from build123d import *

# Parameters (mm, degrees)
ESBO_O1_W                = 8.5
ESBO_O1_H                = 27
RESSALTO_EXTRUS_O1_DEPTH = 13
ESBO_O3_R                = 8.3
CORTE_EXTRUS_O1_DEPTH    = 3
ESBO_O4_R                = 6.3
CORTE_EXTRUS_O2_DEPTH    = 5
ESBO_O7_R                = 8.3
CORTE_EXTRUS_O3_DEPTH    = 0.7
ESBO_O8_R                = 2
CORTE_EXTRUS_O4_DEPTH    = 14


with BuildPart() as part:
    # Esboço1 → Ressalto-extrusão1 (new body)
    with BuildSketch(Plane.XY):
        with Locations((4.75, 202.468429513)):
            Rectangle(ESBO_O1_W, ESBO_O1_H)
    extrude(amount=RESSALTO_EXTRUS_O1_DEPTH)

    # Esboço3 → Corte-extrusão1 (cut)
    with BuildSketch(Plane(origin=(9, 0, 0), x_dir=(0, 0, -1), z_dir=(1, 0, 0))):
        with Locations((0, 202.468429513)):
            Circle(ESBO_O3_R)
    extrude(amount=-CORTE_EXTRUS_O1_DEPTH, mode=Mode.SUBTRACT)

    # Esboço4 → Corte-extrusão2 (cut)
    with BuildSketch(Plane(origin=(6, 0, 0), x_dir=(0, 0, -1), z_dir=(1, 0, 0))):
        with Locations((0, 202.468429513)):
            Circle(ESBO_O4_R)
    extrude(amount=-CORTE_EXTRUS_O2_DEPTH, mode=Mode.SUBTRACT)

    # Esboço7 → Corte-extrusão3 (cut)
    with BuildSketch(Plane.ZY.offset(-0.5)):
        with Locations((0, 202.468429513)):
            Circle(ESBO_O7_R)
    extrude(amount=-CORTE_EXTRUS_O3_DEPTH, mode=Mode.SUBTRACT)

    # Esboço8 → Corte-extrusão4 (cut, through all)
    with BuildSketch(Plane.XY.offset(13)):
        with Locations((4.75, 191.968429513)):
            Circle(ESBO_O8_R)
        with Locations((4.75, 212.968429513)):
            Circle(ESBO_O8_R)
    extrude(amount=-CORTE_EXTRUS_O4_DEPTH, mode=Mode.SUBTRACT)


solid = part.part
Model file for the job. Use its own axes, mm. A direction names the side the tool comes from. Coordinates: 2 decimals unless noted, no trailing zeros. Order: outer loops, then holes, each group sorted by start corner. A loop starts at its lowest first (then second) coordinate and runs counter-clockwise, first axis right, second up. Notation, with made-up numbers: (12.5, -28.75) -> (51.5, -28.75) arc R33 cw to (51.5, 6.25) -> close; hole circle Ø9 at (23.5, -23). An arc over 180 degrees is marked (long way). Return JSON: item names as keys, results as strings. Group by question number.
Item 1: Saw through at B-B on x = 4.75. Write the cut outline in (y, z).
Item 2: Wall check: line 1 along Y through (x, z) = (4.75, 8.5); line 2 along Y through (x, z) = (5.25, 10.5); line 3 along Y through (x, z) = (7, 5.75). Give the ranges that are in metal, low to high. Write a range as [from, to].
Item 3: Saw through at C-C on z = 8. Write the cut outline in (x, y), then the cut area to 3 significant figures.
Item 4: Tool access for faces 4 (the cylindrical face through (0.8, 202.3, 8.3)), 5 (the flat face through (2.8, 193.4, 0)), 6 (the cylindrical face through (7.52, 202.65, 8.3)): list every direction of +Z, -Z, +X, -X, +Y, -Y with a clear straight run to the whole face (end or side of a thin tool).
Item 5: Saw through at A-A on z = 1. Write the cut outline in (x, y), then the cut area to 3 significant figures.
Item 6: Flat gauge pins, fed straight in: P1, Ø4, axis at y = 203, z = 5, coming from the +X side; P2, Ø4, axis at y = 198.5, z = 4.5, coming from the -X side; P3, Ø2.5, axis at x = 4.75, y = 191.97, coming from the -Z side; P4, Ø3, axis at x = 6.5, y = 205, coming from the -Z side. Where does each tip first touch, or does it go through?
Item 7: Saw through at D-D on y = 201.5. Write the cut outline in (x, z).
Item 8: Pull direction X, two halves, no side cores. Call faces 1 (the flat face through (1.2, 203, 7)), 2 (the cylindrical face through (5.673, 190.194, 6.591)), 3 (the flat face through (5, 188.968, 6)): pulls with the +X half, pulls with the -X half, needs draft (parallel to the pull), parting line crosses it, or undercut.
Values found:
{
 "1": {"outline": "(188.97, 0) -> (189.97, 0) -> (189.97, 13) -> (188.97, 13) -> close; (193.97, 0) -> (196.17, 0) arc R6.3 cw to (208.77, 0) -> (210.97, 0) -> (210.97, 13) -> (193.97, 13) -> close; (214.97, 0) -> (215.97, 0) -> (215.97, 13) -> (214.97, 13) -> close"},
 "2": {"line 1": "y = [188.97, 189.97], [193.97, 210.97], [214.97, 215.97]", "line 2": "y = [188.97, 190.03], [193.9, 211.03], [214.9, 215.97]", "line 3": "y = [188.97, 196.48], [208.45, 215.97]"},
 "3": {"outline": "(0.5, 188.97) -> (9, 188.97) -> (9, 200.26) -> (6, 200.26) -> (6, 204.68) -> (9, 204.68) -> (9, 215.97) -> (0.5, 215.97) -> (0.5, 204.68) -> (1.2, 204.68) -> (1.2, 200.26) -> (0.5, 200.26) -> close; hole circle Ø4 at (4.75, 191.97); hole circle Ø4 at (4.75, 212.97)", "area": "188 mm2"},
 "4": {"face 4": "-Z, -X", "face 5": "-Z, +X, -X, +Y, -Y", "face 6": "-Z, +X"},
 "5": {"outline": "(0.5, 188.97) -> (9, 188.97) -> (9, 194.23) -> (6, 194.23) -> (6, 196.25) -> (1.2, 196.25) -> (1.2, 194.23) -> (0.5, 194.23) -> close; (0.5, 210.71) -> (1.2, 210.71) -> (1.2, 208.69) -> (6, 208.69) -> (6, 210.71) -> (9, 210.71) -> (9, 215.97) -> (0.5, 215.97) -> close; hole circle Ø4 at (4.75, 191.97); hole circle Ø4 at (4.75, 212.97)", "area": "83.7 mm2"},
 "6": {"P1": "stops at x = 6", "P2": "stops at x = 1.2", "P3": "passes through", "P4": "stops at z = 4.91"},
 "7": {"outline": "(0.5, 8.24) -> (1.2, 8.24) -> (1.2, 6.23) -> (6, 6.23) -> (6, 8.24) -> (9, 8.24) -> (9, 13) -> (0.5, 13) -> close"},
 "8": {"face 1": "pulls with the -X half", "face 2": "undercut", "face 3": "needs draft"}
}
